The drawing under review shows one solid part. Ordinate dimensions are in mm from its lowest x, y, z. A direction names the side the tool comes from. Coordinates: 2 decimals unless noted, no trailing zeros. Loops run counter-clockwise (first coordinate to the right, second up) from the corner with the lowest first, then second, coordinate; pieces in that order, holes last. Notation, with made-up numbers: (43, 13.5) -> (80, 13.5) arc R19 ccw to (80, 34.5) -> close; hole circle Ø2 at (12, 20). An arc over 180 degrees is marked (long way). Use a Markdown table: item, result.
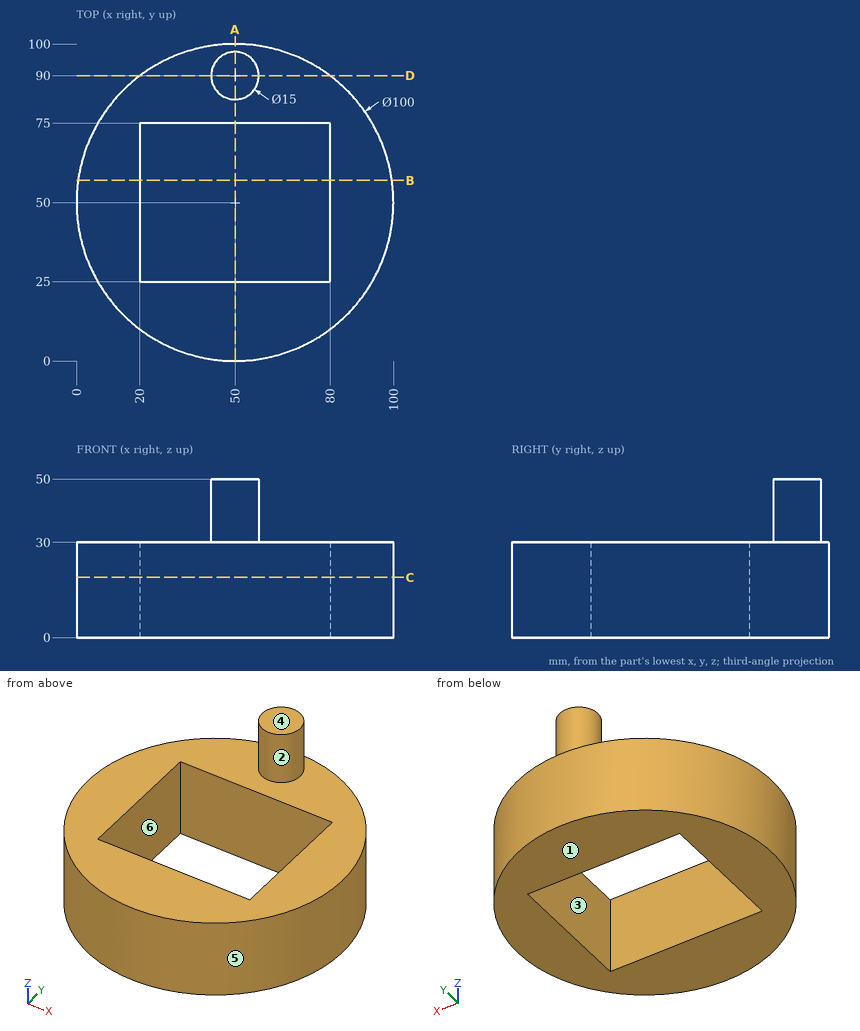
(1) For the marked faces 1, 2 and 3, list the 3-axis set-ups (+Z, -Z, +X, -X, +Y, -Y) from which the entire face can be reached by the end or side of a thin tool; tool diameter is ignored.
Found:
| item | result |
|---|---|
| face 1 | -Z, +X, -X, +Y, -Y |
| face 2 | +Z |
| face 3 | +Z, -Z |
(2) Take a section at B-B on y = 57. Write out the cut boundary in (x, z).
Found:
| item | result |
|---|---|
| outline | (0.49, 0) -> (20, 0) -> (20, 30) -> (0.49, 30) -> close; (80, 0) -> (99.51, 0) -> (99.51, 30) -> (80, 30) -> close |
(3) Take a section at A-A on x = 50. Write out the cut boundary in (y, z), plus the area to 3 significant figures.
Found:
| item | result |
|---|---|
| outline | (0, 0) -> (25, 0) -> (25, 30) -> (0, 30) -> close; (75, 0) -> (100, 0) -> (100, 30) -> (97.5, 30) -> (97.5, 50) -> (82.5, 50) -> (82.5, 30) -> (75, 30) -> close |
| area | 1,800 mm^2 |
(4) Mouldability with a two-part tool opening along X and no side actions: class the marked faces 4, 5 and 6 as pulls with the +X half, pulls with the -X half, needs draft (parallel to the pull), parting line crosses it, or undercut.
Found:
| item | result |
|---|---|
| face 4 | needs draft |
| face 5 | parting line crosses it |
| face 6 | undercut |
(5) For line 1 along Z through (x, y) = (13, 34); line 2 along Y through (x, z) = (36, 13.5); line 3 along Y through (x, z) = (22.5, 28), list the stretches that pass through material, from the lowest coordinate up.
Found:
| item | result |
|---|---|
| line 1 | z = 0 to 30 |
| line 2 | y = 2 to 25, 75 to 98 |
| line 3 | y = 8.24 to 25, 75 to 91.76 |
(6) For pin 1 Ø9 at (x, z) = (63.5, 16.5) entering from +Y; pin 2 Ø9 at (y, z) = (43.5, 20) entering from +X; pin 3 Ø24 at (x, z) = (56, 19.5) entering from -Y; pin 4 Ø6 at (y, z) = (52.5, 34) entering from -X, all flat-tipped, find the tip position at first contact; note any pin that passes through.
Found:
| item | result |
|---|---|
| pin 1 | stops at y = 99.18 |
| pin 2 | stops at x = 99.96 |
| pin 3 | stops at y = 0 |
| pin 4 | passes through |
(7) Take a section at C-C on z = 19. Write out the cut boundary in (x, y), plus the area to 3 significant figures.
Found:
| item | result |
|---|---|
| outline | circle Ø100 at (50, 50); hole (20, 25) -> (80, 25) -> (80, 75) -> (20, 75) -> close |
| area | 4,850 mm^2 |
(8) Take a section at D-D on y = 90. Write out the cut boundary in (x, z), plus the area to 3 significant figures.
Found:
| item | result |
|---|---|
| outline | (20, 0) -> (80, 0) -> (80, 30) -> (57.5, 30) -> (57.5, 50) -> (42.5, 50) -> (42.5, 30) -> (20, 30) -> close |
| area | 2,100 mm^2 |
